```python
from build123d import *

# Parameters (mm, degrees)
EPAISSEUR_PLAQUE_DEPTH          = 2
ESQUISSE5_R                     = 1.75
PERCAGE_FIS_FIXATIONS_DEPTH     = 2
ARRONDIS_EXTREMITES_R           = 4
ESQUISSE10_R                    = 10
ESQUISSE10_R_2                  = 12.5
ESQUISSE10_R_3                  = 11.697835519
EVIDEMENT_DE_MATI_RE_DEPTH      = 2
ESQUISSE11_W                    = 21
ESQUISSE11_H                    = 41
ESQUISSE11_R                    = 2
EMPLACEMENTS_SERVOMOTEURS_DEPTH = 10


with BuildPart() as part:
    # Esquisse3 → Epaisseur plaque (new body)
    with BuildSketch(Plane.XY):
        with BuildLine():
            ThreePointArc((60.676831069, -44.083127967), (0.112789047, 74.999915191), (-60.809145642, -43.900430594))
            ThreePointArc((-60.809145642, -43.900430594), (-0.037511568, -24.943596323), (60.676831069, -44.083127967))
        make_face()
    extrude(amount=EPAISSEUR_PLAQUE_DEPTH)

    # Esquisse5 → Percage fis fixations (cut)
    with BuildSketch(Plane.XY.offset(2)):
        with Locations((0, 70)):
            Circle(ESQUISSE5_R)
        with Locations((60.621778265, -35)):
            Circle(ESQUISSE5_R)
        with Locations((-60.621778265, -35)):
            Circle(ESQUISSE5_R)
    extrude(amount=-PERCAGE_FIS_FIXATIONS_DEPTH, mode=Mode.SUBTRACT)

    # Arrondis extremites
    arrondis_extremites_edges = [part.edges().sort_by_distance(p)[0] for p in [
        (-60.809145642, -43.900430594, 1),
        (60.676831069, -44.083127967, 1),
    ]]
    fillet(arrondis_extremites_edges, radius=ARRONDIS_EXTREMITES_R)

    # Esquisse10 → Evidement de matière (cut)
    with BuildSketch(Plane.XY.offset(2)):
        with Locations((-44.375477733, 40.460370332)):
            Circle(ESQUISSE10_R)
        with Locations((-55.259118801, 17.647943075)):
            Circle(ESQUISSE10_R)
        with Locations((-55.259118801, -9.36594672)):
            Circle(ESQUISSE10_R_2)
        with Locations(Location((55.230698855, -9.532107458, 0), (0, 0, 180))):
            Circle(ESQUISSE10_R_2)
        with Locations(Location((55.311948653, 17.481660149, 0), (0, 0, 180))):
            Circle(ESQUISSE10_R)
        with Locations(Location((44.496969854, 40.326718999, 0), (0, 0, 180))):
            Circle(ESQUISSE10_R)
        with Locations((-19.404495621, 54.872818382)):
            Circle(ESQUISSE10_R_3)
        with Locations(Location((19.569449075, 54.814207195, 0), (0, 0, 180))):
            Circle(ESQUISSE10_R_3)
    extrude(amount=-EVIDEMENT_DE_MATI_RE_DEPTH, mode=Mode.SUBTRACT)

    # Esquisse11 → Emplacements servomoteurs (cut)
    with BuildSketch(Plane.XY.offset(2)):
        Polygon((-1.891789392, 30.96484727), (-2.015105277, -10.03496728), (-23.015010291, -9.971805486), (-22.891694406, 31.028009065), align=None)
        with Locations((12.484913946, 10.459017268)):
            Rectangle(ESQUISSE11_W, ESQUISSE11_H)
        with Locations((7.56186672, 35.974032472)):
            Circle(ESQUISSE11_R)
        with Locations((17.546338474, 35.959017268)):
            Circle(ESQUISSE11_R)
        with Locations((-7.453633256, 35.996613617)):
            Circle(ESQUISSE11_R)
        with Locations((-17.438105011, 36.011628821)):
            Circle(ESQUISSE11_R)
        with Locations((-17.522560101, -14.988347843)):
            Circle(ESQUISSE11_R)
        with Locations((17.477400322, -15.040982732)):
            Circle(ESQUISSE11_R)
        with Locations((7.47741163, -15.025944192)):
            Circle(ESQUISSE11_R)
        with Locations((-7.522571408, -15.003386383)):
            Circle(ESQUISSE11_R)
    extrude(amount=-EMPLACEMENTS_SERVOMOTEURS_DEPTH, mode=Mode.SUBTRACT)


solid = part.part
```
Model file for the job. Use its own axes, mm. Give positions to 0.01 mm unless a question says otherwise; leave off trailing zeros. Order: outer loops, then holes, each group sorted by start corner. A loop starts at its lowest first (then second) coordinate and runs counter-clockwise, first axis right, second up.
1) Wall check: probe 1 along X at (y, z) = (15.5, 1.8); probe 2 along X at (y, z) = (-6.5, 1.6); probe 3 along Y at (x, z) = (-62, 0.95). Give the ranges that are in metal, low to high.
2) Mould opens along Y. For faces 1 (the cylindrical face through (-0.888, -24.946, 0.986)), 2 (the cylindrical face through (-21.94, 43.453, 1.014)), 3 (the flat face through (-1, 17, 2)) say: +Y half, -Y half, draft (parallel to the pull), parting line (faces both ways), or undercut.
3) Saw through at C-C, the plane y = 56.5. Write the cut outline in (x, z).
4) Saw through at A-A, the plane y = 0. Write the cut outline in (x, z).
5) Saw through at D-D, the plane z = 0.45. Count the separate pieces of the cut face and the enclosed holes in it, then the cut area to 3 significant figures.
6) Saw through at B-B, the plane y = 70. Write the cut outline in (x, z), then the cut area to 3 significant figures.
Computed:
1. probe 1: x = -73.38 to -65.03, -45.49 to -22.94, -1.94 to 1.98, 22.98 to 45.51, 65.11 to 73.38
1. probe 2: x = -74.72 to -67.43, -43.09 to -23, -2 to 1.98, 22.98 to 43.1, 67.36 to 74.72
1. probe 3: y = -41.67 to -36.08, -33.92 to -19.89, 1.16 to 10.26, 25.03 to 42.2
2. face 1: -Y half
2. face 2: undercut
2. face 3: draft
3. outline: (-49.32, 0) - (-30.99, 0) - (-30.99, 2) - (-49.32, 2) - close; (-7.82, 0) - (7.99, 0) - (7.99, 2) - (-7.82, 2) - close; (31.15, 0) - (49.32, 0) - (49.32, 2) - (31.15, 2) - close
4. outline: (-75, 0) - (-63.54, 0) - (-63.54, 2) - (-75, 2) - close; (-46.98, 0) - (-22.99, 0) - (-22.99, 2) - (-46.98, 2) - close; (-1.98, 0) - (1.98, 0) - (1.98, 2) - (-1.98, 2) - close; (22.98, 0) - (47.14, 0) - (47.14, 2) - (22.98, 2) - close; (63.32, 0) - (75, 0) - (75, 2) - (63.32, 2) - close
5. separate pieces: 1
5. enclosed holes: 21
5. area: 8,500 mm2
6. outline: (-26.93, 0) - (-1.75, 0) - (-1.75, 2) - (-26.93, 2) - close; (1.75, 0) - (26.93, 0) - (26.93, 2) - (1.75, 2) - close
6. area: 101 mm2
